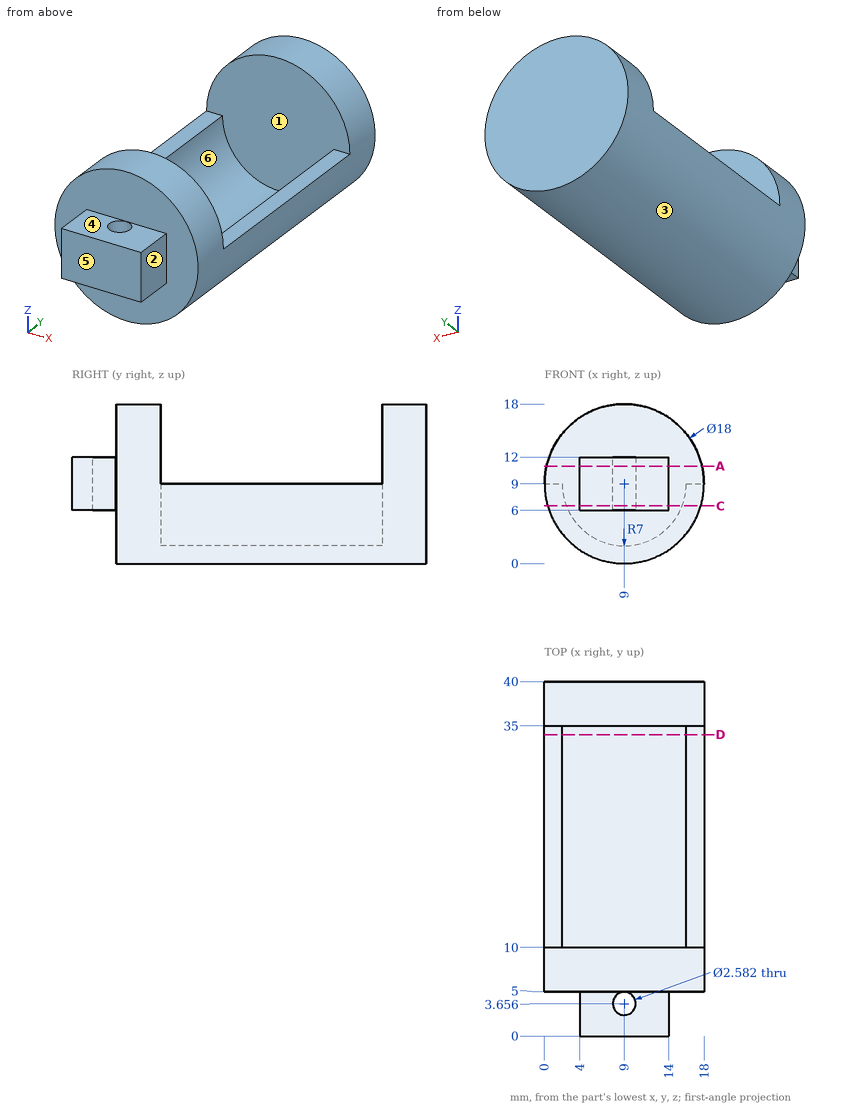
Check sheet for the drawn part. Datum: minimum x, y, z corner. Units: mm. A direction names the side the tool comes from. Give positions to 0.01 mm unless a question says otherwise; leave off trailing zeros. Loops run counter-clockwise (first coordinate to the right, second up) from the corner with the lowest first, then second, coordinate; pieces in that order, holes last.
1) Sectioned sample at A-A, the plane z = 11. Enter the section's corners in (x, y) (1 decimal), then the cut area to 3 significant figures.
2) Sectioned sample at C-C, the plane z = 6.5. Enter the section's corners in (x, y) (1 decimal).
3) Draft check along X on the marked faces 1, 2, 3 and 4. Enter one of: pulls with the +X half, pulls with the -X half, needs draft (parallel to the pull), parting line crosses it, or undercut.
4) Depth check by flat-ended pin: pin 1 Ø1.5 at (x, y) = (10.5, 1.5) entering from -Z; pin 2 Ø2.5 at (y, z) = (2, 9.5) entering from -X; pin 3 Ø5 at (x, y) = (8.5, 26.5) entering from +Z (1 decimal); pin 4 Ø8 at (x, z) = (13, 9.5) entering from -Y. Enter the tip coordinate at first touch or a pass-through.
5) Set-up check for the marked faces 5 and 6: record each of +Z, -Z, +X, -X, +Y, -Y from which the full face is reachable in a straight line by a thin tool's end or side.
6) Thickness scan on line 1 along Y through (x, z) = (9, 8.15) (1 decimal); line 2 along Y through (x, z) = (9.5, 16.25); line 3 along Y through (x, z) = (1.25, 6.5). Record the ranges inside material, lowest first.
7) Sectioned sample at D-D, the plane y = 34. Enter the section's corners in (x, z).
Answers:
1. outline: (0.2, 5) - (4, 5) - (4, 0) - (14, 0) - (14, 5) - (17.8, 5) - (17.8, 10) - (0.2, 10) - close; (0.2, 35) - (17.8, 35) - (17.8, 40) - (0.2, 40) - close; hole circle Ø2.6 at (9, 3.7)
1. area: 220 mm2
2. outline: (0.4, 5) - (4, 5) - (4, 0) - (14, 0) - (14, 5) - (17.6, 5) - (17.6, 40) - (0.4, 40) - close; hole (2.5, 10) - (15.5, 10) - (15.5, 35) - (2.5, 35) - close; hole circle Ø2.6 at (9, 3.7)
3. face 1: undercut
3. face 2: pulls with the +X half
3. face 3: parting line crosses it
3. face 4: needs draft
4. pin 1: stops at z = 6
4. pin 2: stops at x = 4
4. pin 3: stops at z = 2.7
4. pin 4: stops at y = 0
5. face 5: +Z, -Z, +X, -X, -Y
5. face 6: +Z
6. line 1: y = 0 to 2.4, 4.9 to 10, 35 to 40
6. line 2: y = 5 to 10, 35 to 40
6. line 3: y = 5 to 40
7. outline: (0, 9) arc R9 ccw to (18, 9) - (16, 9) arc R7 cw to (2, 9) - close
